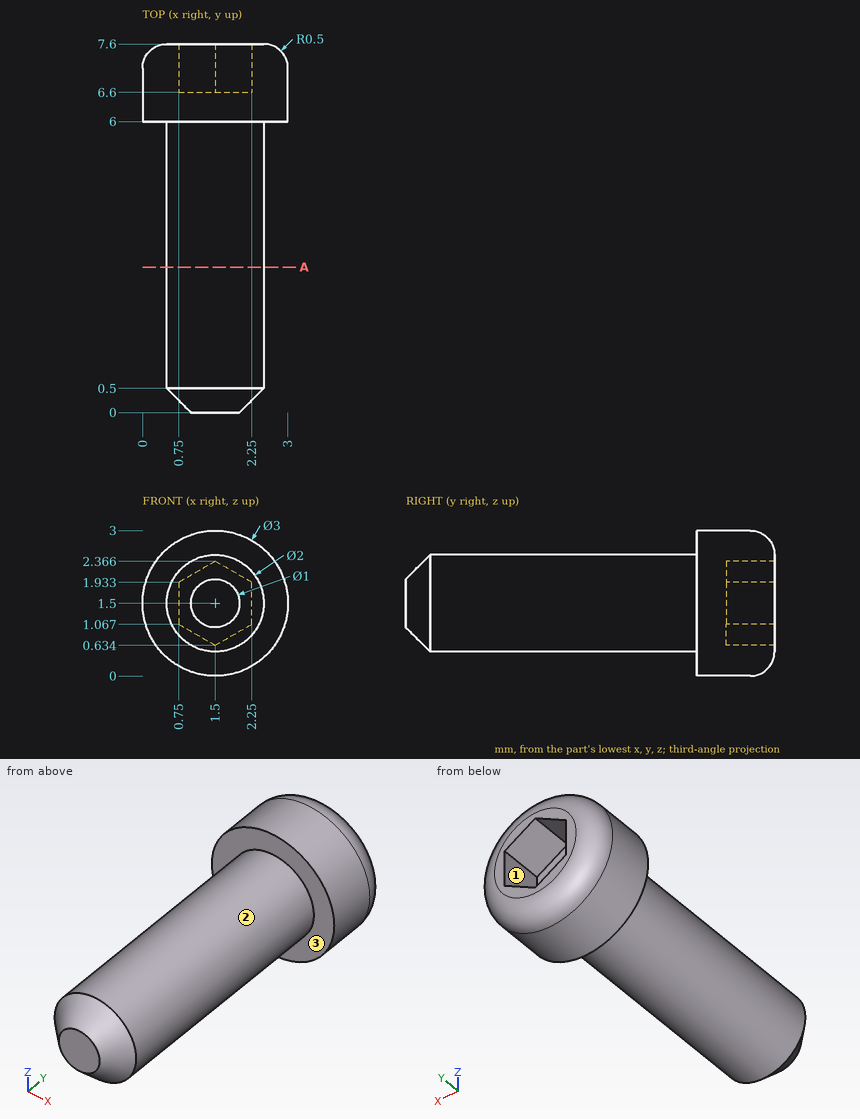
Verification items for this drawing (mm, ordinates from the low corner). Give positions to 0.01 mm unless a question says otherwise; leave off trailing zeros. Loops run counter-clockwise (first coordinate to the right, second up) from the corner with the lowest first, then second, coordinate; pieces in that order, holes last. Notation, with made-up numbers: M -2.5,82 L 56.5,82 A28 cw 56.5,102 Z; hole C 23,-8 d11. An arc over 180 degrees is marked long. Answer in a Markdown table with one row per item.
1) Thickness scan on line 1 (X direction, y = 4.5, z = 2.4); line 2 (Y direction, x = 1.9, z = 1.6); line 3 (Z direction, x = 1.3, y = 0.75). Record the ranges inside material, lowest first.
Solutions:
| item | result |
|---|---|
| line 1 | x = 1.06 to 1.94 |
| line 2 | y = 0 to 6.6 |
| line 3 | z = 0.52 to 2.48 |
2) Depth check by flat-ended pin: pin 1 (1.5 mm diameter, centred on y = 3.5, z = 0.5, fed in from -X); pin 2 (1.2 mm diameter, centred on x = 1.5, z = 1, fed in from +Y); pin 3 (1 mm diameter, centred on x = 0.5, z = 2, fed in from -Y). Enter the tip coordinate at first touch or a pass-through.
Solutions:
| item | result |
|---|---|
| pin 1 | stops at x = 0.53 |
| pin 2 | stops at y = 7.6 |
| pin 3 | stops at y = 0.12 |
3) Cross-section at A-A (y = 3). Enter the section's corners in (x, z), plus the area to 3 significant figures.
Solutions:
| item | result |
|---|---|
| outline | C 1.5,1.5 d2 |
| area | 3.14 mm^2 |
4) Mould release check, pull along Z, two halves, no side actions. Record for the marked faces 1, 2 and 3: released by +Z, released by -Z, zero draft, split by the parting line, or undercut.
Solutions:
| item | result |
|---|---|
| face 1 | undercut |
| face 2 | split by the parting line |
| face 3 | zero draft |
